from build123d import *

# Parameters (mm, degrees)
SKETCH2_R           = 6.9
BOSS_EXTRUDE1_DEPTH = 3
SKETCH3_R           = 6.9
SKETCH3_R_2         = 5
BOSS_EXTRUDE2_DEPTH = 13
CHAMFER1_SIZE       = 0.5
CHAMFER2_SIZE       = 1
SKETCH4_R           = 1.375
CUT_EXTRUDE1_DEPTH  = 20


with BuildPart() as part:
    # Sketch2 → Boss-Extrude1 (new body)
    with BuildSketch(Plane.XY):
        with BuildLine():
            Line((102.765440341, 138.860814374), (120.765440341, 138.860814374))
            ThreePointArc((120.765440341, 138.860814374), (121.472547122, 138.567921155), (121.765440341, 137.860814374))
            Line((121.765440341, 137.860814374), (121.765440341, 118.860814374))
            ThreePointArc((121.765440341, 118.860814374), (120.300974247, 115.325280468), (116.765440341, 113.860814374))
            Line((116.765440341, 113.860814374), (106.765440341, 113.860814374))
            ThreePointArc((106.765440341, 113.860814374), (103.229906435, 115.325280468), (101.765440341, 118.860814374))
            Line((101.765440341, 118.860814374), (101.765440341, 137.860814374))
            ThreePointArc((101.765440341, 137.860814374), (102.058333559, 138.567921155), (102.765440341, 138.860814374))
        make_face()
        with Locations((111.765440341, 128.860814374)):
            Circle(SKETCH2_R, mode=Mode.SUBTRACT)
    extrude(amount=BOSS_EXTRUDE1_DEPTH)

    # Sketch3 → Boss-Extrude2 (add)
    with BuildSketch(Plane.XY):
        with Locations(Location((111.765440341, 128.860814374, 0), (0, 0, 180))):
            Circle(SKETCH3_R)
        with Locations(Location((111.765440341, 128.860814374, 0), (0, 0, 180))):
            Circle(SKETCH3_R_2, mode=Mode.SUBTRACT)
    extrude(amount=BOSS_EXTRUDE2_DEPTH)

    # Chamfer1
    chamfer1_edges = [part.edges().sort_by_distance(p)[0] for p in [
        (121.472547122, 138.567921155, 0),
        (121.765440341, 128.360814374, 0),
        (111.765440341, 138.860814374, 3),
        (120.300974247, 115.325280468, 0),
        (111.765440341, 113.860814374, 0),
        (103.229906435, 115.325280468, 0),
        (101.765440341, 128.360814374, 0),
        (102.058333559, 138.567921155, 0),
        (111.765440341, 138.860814374, 0),
        (102.058333559, 138.567921155, 3),
        (101.765440341, 128.360814374, 3),
        (103.229906435, 115.325280468, 3),
        (118.665440341, 128.860814374, 13),
        (116.765440341, 128.860814374, 0),
        (116.765440341, 128.860814374, 13),
        (111.765440341, 113.860814374, 3),
        (120.300974247, 115.325280468, 3),
        (121.765440341, 128.360814374, 3),
        (121.472547122, 138.567921155, 3),
    ]]
    chamfer(chamfer1_edges, length=CHAMFER1_SIZE)

    # Chamfer2
    chamfer2_edges = [part.edges().sort_by_distance(p)[0] for p in [
        (118.665440341, 128.860814374, 3),
    ]]
    chamfer(chamfer2_edges, length=CHAMFER2_SIZE)

    # Sketch4 → Cut-Extrude1 (cut)
    with BuildSketch(Plane(origin=(0, 138.860814374, 0), x_dir=(1, 0, 0), z_dir=(0, 1, 0))):
        with Locations(Location((112.244247242, -8.875, 0), (0, 0, 270))):
            Circle(SKETCH4_R)
    extrude(amount=-CUT_EXTRUDE1_DEPTH, mode=Mode.SUBTRACT)


solid = part.part
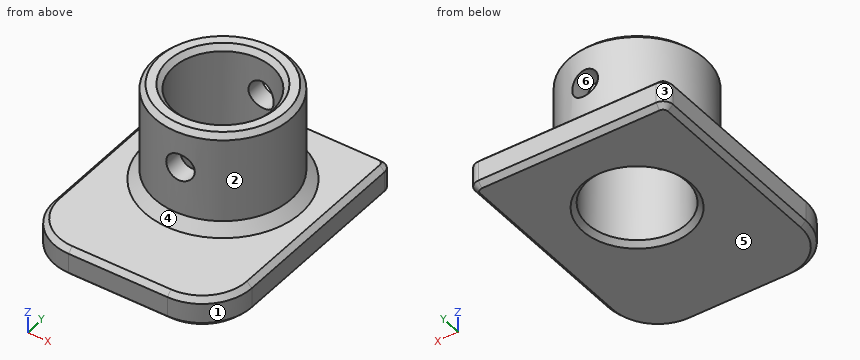
Verification items for the finished model (mm, model axes). Face numbers are marked on the shaded views. A direction names the side the tool comes from. Coordinates: 2 decimals unless noted, no trailing zeros. Order: outer loops, then holes, each group sorted by start corner. A loop starts at its lowest first (then second) coordinate and runs counter-clockwise, first axis right, second up. Notation, with made-up numbers: M -23,-21 L 30,-21 A29 ccw 30,3 Z; hole C 49,50 d2. An arc over 180 degrees is marked long. Return JSON: item names as keys, results as strings.
1) Cross-section at A-A, the plane z = 3.5. Record the boundary of the cut face in (x, y).
Answer list:
{"outline": "C 111.77,128.86 d14.8; hole C 111.77,128.86 d10"}
2) Release check for a two-part mould opening along X. For the marked faces 3, 4, 5 and 6 record: +X half, -X half, draft (parallel to the pull), parting line (faces both ways), or undercut.
Answer list:
{"face 3": "-X half", "face 4": "parting line", "face 5": "draft", "face 6": "undercut"}
3) Cross-section at B-B, the plane x = 111.5. Count the separate pieces of the cut face and the enclosed holes in it, and give its area (3 significant figures).
Answer list:
{"separate pieces": "4", "enclosed holes": "0", "area": "74.0 mm2"}
4) Access from +Z, -Z, +X, -X, +Y, -Y to the whole of each face (thin tool, end or side, straight path). Record for the marked faces 1 and 2.
Answer list:
{"face 1": "+Z, -Z, +X, -Y", "face 2": "+Z"}
5) Gauge pin test, flat ends, axial feed: pin 1 (4 mm diameter, centred on x = 110.5, z = 6.5, fed in from -Y); pin 2 (1.6 mm diameter, centred on x = 112.24, z = 8.88, fed in from -Y); pin 3 (5 mm diameter, centred on y = 131, z = 3, fed in from +X); pin 4 (3 mm diameter, centred on x = 117, z = 10.5, fed in from -Y). Record the tip position at first contact, or that the pin passes through.
Answer list:
{"pin 1": "y = 121.96", "pin 2": "through", "pin 3": "x = 121.77", "pin 4": "y = 123.06"}
6) Thickness scan on L1, parallel to Z at x = 121, y = 121; L2, parallel to X at y = 126.75, z = 12; L3, parallel to Y at x = 110.75, z = 5.5. Record the ranges inside material, lowest first. Write a range as [from, to].
Answer list:
{"L1": "[0, 3]", "L2": "[105.2, 107.23], [116.3, 118.33]", "L3": "[122.04, 123.97], [133.76, 135.69]"}
